Print and shaded views of the part. All mm, measured from the part's lowest x, y and z. A direction names the side the tool comes from. Coordinates: 2 decimals unless noted, no trailing zeros. Order: outer loops, then holes, each group sorted by start corner. A loop starts at its lowest first (then second) coordinate and runs counter-clockwise, first axis right, second up.
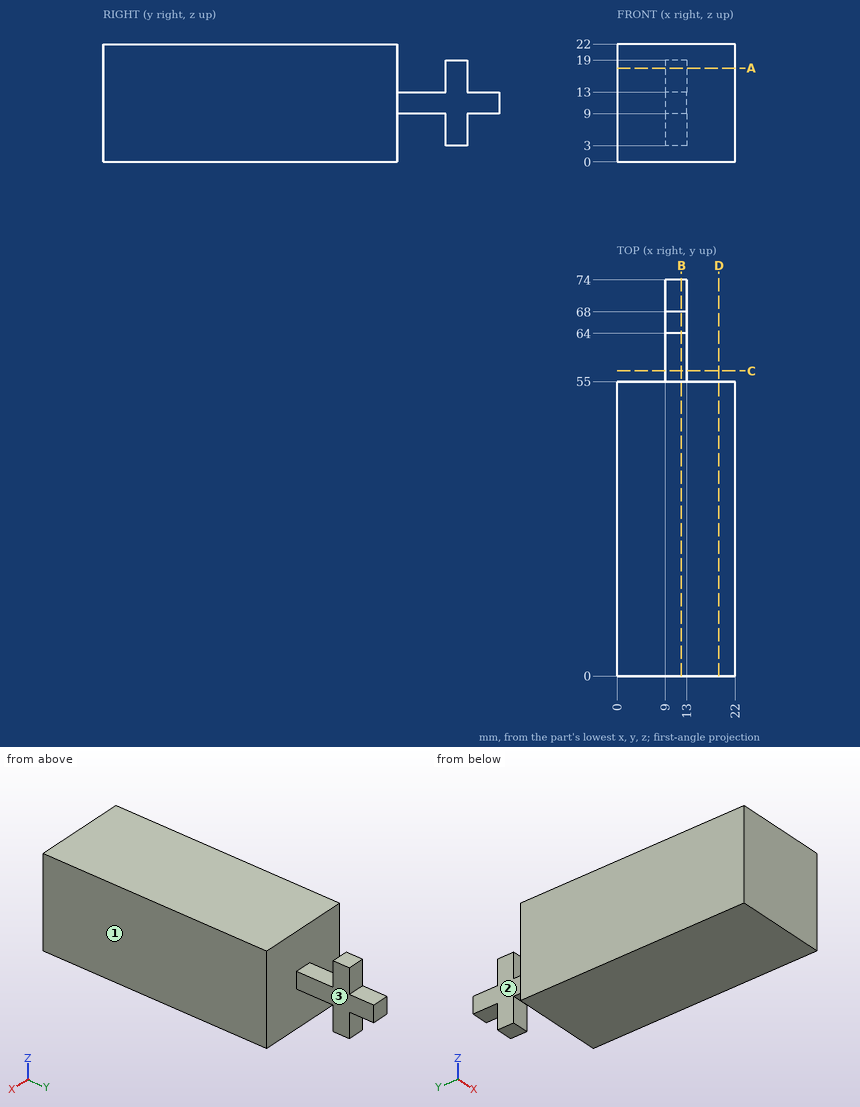
Q1. Cut at C-C, the plane y = 57. List the corners of the cut face in (x, z), plus the area to 3 significant figures.
Established:
outline: (9, 9) - (13, 9) - (13, 13) - (9, 13) - close
area: 16.0 mm2
Q2. Cut at B-B, the plane x = 12. List the corners of the cut face in (y, z).
Established:
outline: (0, 0) - (55, 0) - (55, 9) - (64, 9) - (64, 3) - (68, 3) - (68, 9) - (74, 9) - (74, 13) - (68, 13) - (68, 19) - (64, 19) - (64, 13) - (55, 13) - (55, 22) - (0, 22) - close
Q3. Cut at D-D, the plane x = 19. List the corners of the cut face in (y, z), plus the area to 3 significant figures.
Established:
outline: (0, 0) - (55, 0) - (55, 22) - (0, 22) - close
area: 1,210 mm2
Q4. Cut at A-A, the plane z = 17.5. List the corners of the cut face in (x, y).
Established:
outline: (0, 0) - (22, 0) - (22, 55) - (0, 55) - close; (9, 64) - (13, 64) - (13, 68) - (9, 68) - close
Q5. Which spindle directions (+Z, -Z, +X, -X, +Y, -Y) get a long thin tool onto all of the face, cutting with end or side? Do the marked faces 1, 2 and 3. Say none if no direction does.
Established:
face 1: +Z, -Z, +X, +Y, -Y
face 2: +Z, -Z, -X, +Y
face 3: +Z, -Z, +X, +Y
Q6. Probe line 1 (Y direction, x = 12.25, z = 14.25); line 2 (Y direction, x = 7.75, z = 1.5). List the from-to ranges inside material, lowest first.
Established:
line 1: y = 0 to 55, 64 to 68
line 2: y = 0 to 55
Q7. Drop flat-ended pins along their axis: P1, Ø3, axis at x = 11.5, z = 6, coming from the +Y side; P2, Ø3, axis at x = 11.5, y = 72.5, coming from the +Z side; P3, Ø5, axis at y = 63, z = 7, coming from the -X side. Give the stop position or say it passes through.
Established:
P1: stops at y = 68
P2: stops at z = 13
P3: stops at x = 9
